Design review of the part built by this model. Coordinates are the model's own, in mm. Round coordinates to 2 decimals unless told otherwise and drop trailing zeros. Use CSV: the item, a comma, the result in double quotes.
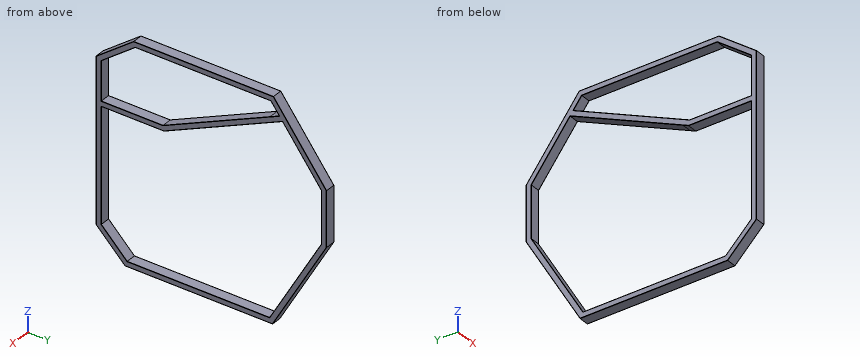
from build123d import *

# Parameters (mm, degrees)
BOSS_EXTRU_1_DEPTH = 80
COQUE1_START       = 4
COQUE1_DEPTH       = 72
CONG_2_R           = 2


# Read off the part's stored shape, not the designer's step: Coque1
with BuildPart() as part:
    # Esquisse1 → Boss.-Extru.1 (new body)
    with BuildSketch(Plane(origin=(0, 0, 0), x_dir=(0, 0, -1), z_dir=(1, 0, 0))):
        Polygon((740, 183.431457505), (740, 1323.212901419), (10.622577483, 1740), (-413.333333333, 1740), (-840, 1420), (-960, 1330), (-960, 250), (-740.540540541, -40), (-419.892357873, -40), (0, -40), (516.568542495, -40), align=None)
        Polygon((-420, 476.25814746), (-420, 26.428571429), (-420, 0), (-450.162628143, 0), (-554.571588527, 0), (-720.648182668, 0), (-920, 263.429187189), (-920, 1310), (-832.74112038, 1375.444159715), (-800, 1304.115290317), align=None, mode=Mode.SUBTRACT)
        Polygon((500, 0), (0, 0), (-380, 0), (-380, 485), (-400, 528.571428571), (-800, 1400), (-400, 1700), (0, 1700), (700, 1300), (700, 200), align=None, mode=Mode.SUBTRACT)
    extrude(amount=BOSS_EXTRU_1_DEPTH)

    # Coque1 outline → Coque1 (cut)
    with BuildSketch(Plane.YZ.offset(COQUE1_START)):
        Polygon((1736, -9.560319735), (1736, 412), (1328, 956), (251.342918719, 956), (-36, 738.551304753), (-36, -514.911688245), (185.088311755, -736), (1320.891611277, -736), align=None)
        Polygon((484.125814746, 384), (1401.263928167, 804.981429111), (1704, 401.333333333), (1704, -1.062257748), (1302.321290142, -704), (198.343145751, -704), (-4, -501.656854249), (-4, 384), align=None, mode=Mode.SUBTRACT)
        Polygon((262.08626847, 924), (1312, 924), (1381.619255939, 831.174325415), (477.132332714, 416), (-4, 416), (-4, 722.637418455), align=None, mode=Mode.SUBTRACT)
    extrude(amount=COQUE1_DEPTH, mode=Mode.SUBTRACT)

    # Congé2
    cong_2_edges = [part.edges().sort_by_distance(p)[0] for p in [
        (80, 942.5, 590),
        (80, 1550, 600),
        (80, 1700, 200),
        (0, 786.714593595, 920),
        (0, 131.714593595, 820.324091334),
        (80, 1500, -350),
        (0, 0, 570.324091334),
        (0, 238.12907373, 420),
        (0, 925.851153588, 626.37056019),
        (0, 1342.722079858, 876.37056019),
        (0, 1740, 201.355377925),
        (0, 1531.606450709, -375.311288741),
        (0, 753.322179462, -740),
        (80, 750, -700),
        (0, 71.715728753, -628.284271247),
        (0, -40, 111.985999023),
        (0, 105, 850.27027027),
        (0, 790, 960),
        (0, 1535, 686.666666667),
        (0, 0, -60),
        (0, 100, -600),
        (80, 100, -600),
        (0, 750, -700),
        (0, 1500, -350),
        (0, 1700, 200),
        (0, 1550, 600),
        (0, 942.5, 590),
        (0, 242.5, 380),
        (80, 0, -60),
        (80, 1535, 686.666666667),
        (80, 790, 960),
        (80, 105, 850.27027027),
        (80, -40, 111.985999023),
        (80, 71.715728753, -628.284271247),
        (80, 753.322179462, -740),
        (80, 1531.606450709, -375.311288741),
        (80, 242.5, 380),
        (76, 1346.80962797, 877.587162708),
        (4, 929.375794326, 623.587162708),
        (76, 236.566166357, 416),
        (76, -4, 569.318709227),
        (80, 1740, 201.355377925),
        (76, 129.043134235, 823.318709227),
        (76, 1532, 684),
        (76, 789.671459359, 956),
        (76, 107.67145936, 847.275652377),
        (76, -36, 111.819808254),
        (4, 74.544155878, -625.455844123),
        (76, 752.989961516, -736),
        (76, 1528.445805639, -372.780159868),
        (76, 240.062907373, 384),
        (76, 942.694871456, 594.490714556),
        (76, 1552.631964083, 603.157381222),
        (4, 1704, 200.135537793),
        (4, 1503.160645071, -352.531128874),
        (4, 750.332217947, -704),
        (76, 97.171572876, -602.828427124),
        (76, 1736, 201.219840132),
        (76, -4, -58.828427125),
        (76, 787.043134235, 924),
        (76, 1704, 200.135537793),
        (76, 1503.160645071, -352.531128874),
        (76, 750.332217947, -704),
        (76, 74.544155878, -625.455844123),
        (80, 1342.722079858, 876.37056019),
        (76, 929.375794326, 623.587162708),
        (4, 240.062907373, 384),
        (4, -4, -58.828427125),
        (4, 97.171572876, -602.828427124),
        (4, 1552.631964083, 603.157381222),
        (4, 942.694871456, 594.490714556),
        (4, 1532, 684),
        (4, 1736, 201.219840132),
        (4, 1528.445805639, -372.780159868),
        (4, 752.989961516, -736),
        (4, -36, 111.819808254),
        (4, 107.67145936, 847.275652377),
        (4, 789.671459359, 956),
        (4, 1346.80962797, 877.587162708),
        (4, 787.043134235, 924),
        (4, 129.043134235, 823.318709227),
        (4, -4, 569.318709227),
        (4, 236.566166357, 416),
        (80, 925.851153588, 626.37056019),
        (80, 238.12907373, 420),
        (80, 0, 570.324091334),
        (80, 131.714593595, 820.324091334),
        (80, 786.714593595, 920),
    ]]
    fillet(cong_2_edges, radius=CONG_2_R)


solid = part.part
1) We need section A-A (z = 132). Give the number of separate pieces and of enclosed holes in the cut face, then the cut area to 3 significant figures.
Data:
separate pieces,"2"
enclosed holes,"2"
area,"1,790 mm2"
2) Insertion check: pin 1 Ø10 at (x, y) = (71.5, 1430) entering from -Z; pin 2 Ø23 at (x, z) = (42.5, 640) entering from +Y (3 decimals); pin 3 Ø20.5 at (x, y) = (48.5, 174.5) entering from +Z. Each pin has a flat end and moves straight along its axis. Give the tip position at first contact, or say it passes through.
Data:
pin 1,"stops at z = -561.87"
pin 2,"stops at y = 1578.625"
pin 3,"stops at z = 910.62"
3) To check wall thickness, follow L1, parallel to Z at x = 71, y = 350; L2, parallel to Y at x = 73, z = 35.5; L3, parallel to Y at x = 20, z = 644.5 (3 decimals). State the ranges of each line that lie inside material, in increasing order. Write a range as from..to.
Data:
L1,"z = -740..-736, -704..-700, 380..384, 416..420, 920..924, 956..960"
L2,"y = -40..-36, -4..0, 1700..1704, 1736..1740"
L3,"y = -40..-36, -4..0, 965.347..974.936, 1051.644..1061.232, 1516.625..1521.625, 1561.625..1566.625"
